Check sheet for the modelled part. Datum: model origin and axes. Units: mm. Coordinates: 2 decimals unless noted, no trailing zeros. Write each loop counter-clockwise with the first axis right and the second up, starting at its lowest first coordinate (ties: lowest second). Pieces come first, ordered by that corner, then holes. Notation, with made-up numbers: M -12,11.5 L 28,11.5 A18 ccw 28,28.5 Z; hole C 62.5,3.5 d4. An arc over 180 degrees is marked long. Answer as CSV lines item,"result". Start each with the question number.
1) Material ranges on L1, parallel to X at y = 2.6, z = 0; L2, parallel to X at y = 2, z = 12; L3, parallel to Z at x = 22, y = 0.2, recorded low to high. Write a range as [from, to].
2) Section check B-B (y = 1.5). State how many separate pieces and enclosed holes the cut face has, and give its area (3 significant figures).
3) Go/stop test with flat-tipped pins: pin 1 Ø1 at (x, y) = (13, 0.5) entering from -Z; pin 2 Ø1.5 at (y, z) = (1, -0.5) entering from +X; pin 3 Ø1 at (x, y) = (-8.5, 2) entering from -Z; pin 4 Ø2 at (y, z) = (1, 9.5) entering from -X. Record where each tip stops, or that it passes through.
4) Section check C-C (z = -8). Record the cut outline in (x, y).
5) Section check A-A (x = 0). Record the cut outline in (y, z).
6) Section check D-D (x = -8.5). Record the cut outline in (y, z).
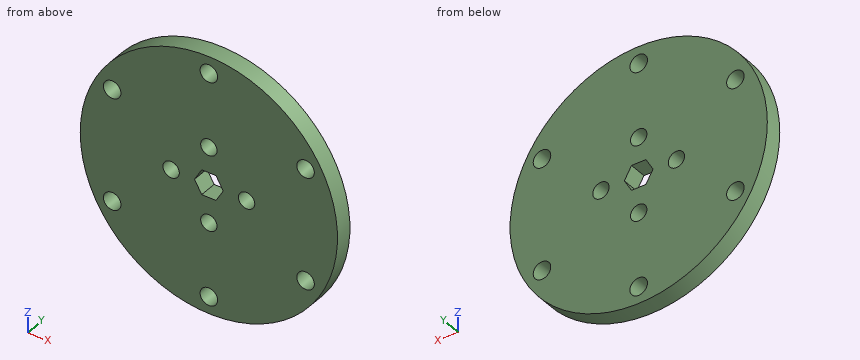
Autodesk Inventor part; units mm, degrees
ref_plane "Work Plane5" through (0, 21.082, 0) normal (0, 1, 0) x (1, 0, 0)
ref_plane "Work Plane6" through (0, 21.082, 0) normal (0, 1, 0) x (1, 0, 0)
ref_plane "YZ Plane" through (0, 0, 0) normal (1, 0, 0) x (0, 1, 0)
sketch "Sketch1" plane through (0, 0, 0) normal (0, 1, 0) x (-1, 0, 0)
  circle A0 centre (0, 0) radius 27.94
  dimension "d0" = 55.88
extrude "Extrusion1" add sketch "Sketch1" along normal blind 7.62
ref_plane "Work Plane5" through (0, 21.082, 0) normal (0, 1, 0) x (1, 0, 0)
sketch "Sketch5" plane through (0, 21.082, 0) normal (0, 1, 0) x (1, 0, 0)
  line L0 (0, 0) -> (0, 2.667)
  line L1 (-3.1168, 0) -> (-1.5584, 2.6992)
  line L2 (-1.5584, 2.6992) -> (1.5584, 2.6992)
  line L3 (1.5584, 2.6992) -> (3.1168, 0)
  line L4 (3.1168, 0) -> (1.5584, -2.6992)
  line L5 (1.5584, -2.6992) -> (-1.5584, -2.6992)
  line L6 (-1.5584, -2.6992) -> (-3.1168, 0)
  dimension "d10" = 2.667
extrude "Extrusion4" cut sketch "Sketch5" against normal blind 25.4
sketch "Sketch6" plane through (0, 7.62, 0) normal (0, 1, 0) x (1, 0, 0)
  circle A0 centre (0, 0) radius 27.94
  line L0 (0, -27.94) -> (0, -26.162)
  line L1 (0, -26.162) -> (0, -24.257)
  circle A1 centre (0, -24.257) radius 1.905
  dimension "d13" = 1.778
  dimension "d14" = 1.905
extrude "Extrusion5" cut sketch "Sketch6" against normal blind 25.4 contours A1
ref_plane "Work Plane6" through (0, 21.082, 0) normal (0, 1, 0) x (1, 0, 0)
pattern_circular "Circular Pattern1" count 6 over 360 about axis through (0, 21.082, 0) along (0, 1, 0) of "Extrusion5"
sketch "Sketch8" plane through (0, 0, 0) normal (0, -1, 0) x (1, 0, 0)
  line L0 (3.1168, 0) -> (1.5584, -2.6992)
  line L1 (3.1168, 0) -> (6.4188, 0)
  line L2 (6.4188, 0) -> (8.1968, 0)
  circle A0 centre (8.1968, 0) radius 1.778
  point P0 (0, 0)
  dimension "d20" = 3.302
  dimension "d21" = 1.778
extrude "Extrusion6" cut sketch "Sketch8" against normal blind 25.4
pattern_circular "Circular Pattern2" count 4 over 360 about axis through (0, 21.082, 0) along (0, 1, 0) of "Extrusion6"
sketch "Sketch10" plane through (0, 7.62, 0) normal (0, 1, 0) x (1, 0, 0)
  circle A0 centre (0, 0) radius 27.94
extrude "Extrusion8" cut sketch "Sketch10" against normal blind 3.81
properties part number "Wheel Mount"
Results found:
1,L1,"x = [-27.94, -9.97], [-6.42, -3.12], [3.12, 6.42], [9.97, 27.94]"
1,L2,"x = [-25.23, -22.91], [-19.11, 19.11], [22.91, 25.23]"
1,L3,"z = [-17.22, -13.75], [-10.5, 10.5], [13.75, 17.22]"
2,separate pieces,"1"
2,enclosed holes,"11"
2,area,"2,320 mm2"
3,pin 1,"stops at z = -24.99"
3,pin 2,"stops at x = 27.94"
3,pin 3,"stops at z = -26.77"
3,pin 4,"stops at x = -26.62"
4,outline,"M -26.77,0 L -1.77,0 L -1.77,3.81 L -26.77,3.81 Z; M 1.77,0 L 26.77,0 L 26.77,3.81 L 1.77,3.81 Z"
5,outline,"M 0,-27.94 L 3.81,-27.94 L 3.81,-26.16 L 0,-26.16 Z; M 0,-22.35 L 3.81,-22.35 L 3.81,-9.97 L 0,-9.97 Z; M 0,-6.42 L 3.81,-6.42 L 3.81,-2.7 L 0,-2.7 Z; M 0,2.7 L 3.81,2.7 L 3.81,6.42 L 0,6.42 Z; M 0,9.97 L 3.81,9.97 L 3.81,22.35 L 0,22.35 Z; M 0,26.16 L 3.81,26.16 L 3.81,27.94 L 0,27.94 Z"
6,outline,"M 0,-26.62 L 3.81,-26.62 L 3.81,-1.75 L 0,-1.75 Z; M 0,1.75 L 3.81,1.75 L 3.81,26.62 L 0,26.62 Z"
